Here's the drawing with two shaded views (mm, measured from the low corner). I have some questions. Coordinates: 2 decimals unless noted, no trailing zeros. Write each loop counter-clockwise with the first axis right and the second up, starting at its lowest first coordinate (ties: lowest second). Pieces come first, ordered by that corner, then holes. Notation, with made-up numbers: (51, -32) -> (75, -32) arc R31 ccw to (75, -7) -> close; hole circle Ø5 at (-19, -30). An arc over 180 degrees is marked (long way). Put each result on its own line as item: value. Start each with the question number.
Item 1: I need wall thicknesses on line 1 (Z direction, x = 6.35, y = 0.9); line 2 (X direction, y = 0.85, z = 107.95); line 3 (Z direction, x = 5.5, y = 1.3) (1 decimal). Which ranges of each line are inside material? Lowest first, please. Write a range as [from, to].
Item 2: I want a section at A-A, the plane x = 6.35. List the corners of the cut face in (y, z) for me.
Item 3: I want a section at B-B, the plane z = 107.95. List the corners of the cut face in (x, y) for me.
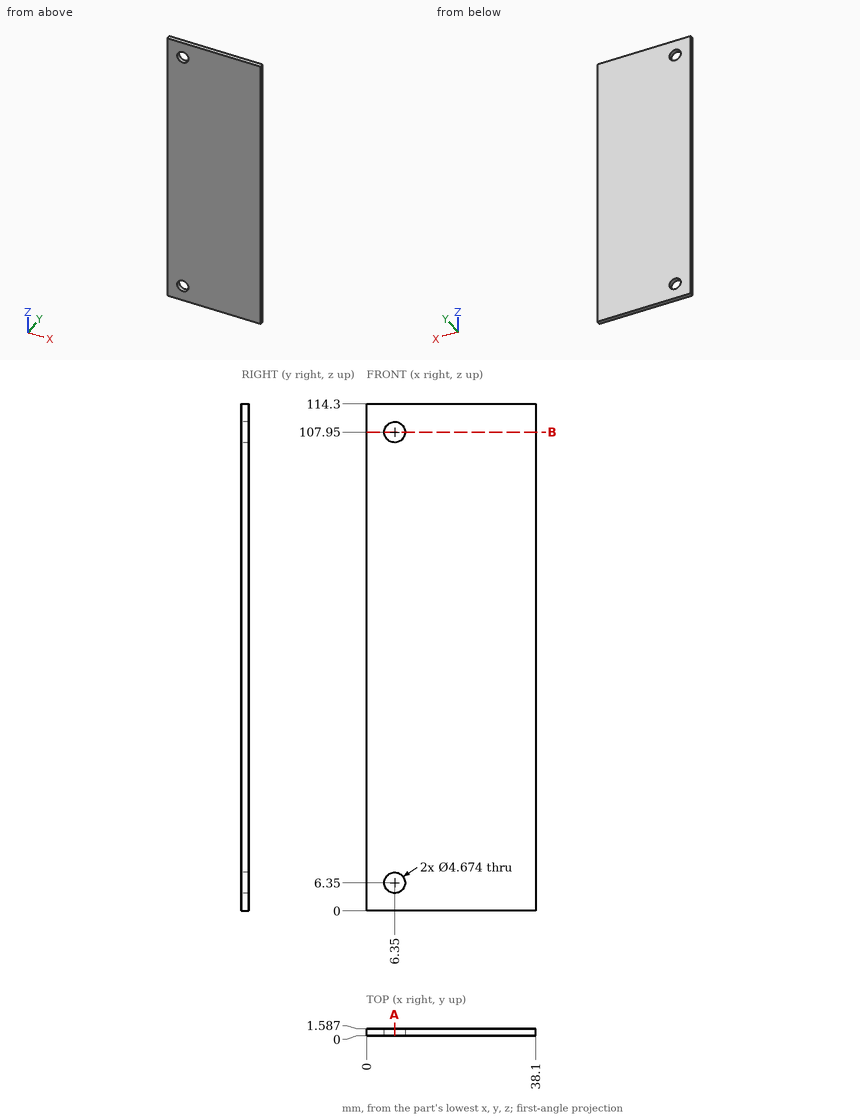
Calculated:
1. line 1: z = [0, 4.01], [8.69, 105.61], [110.29, 114.3]
1. line 2: x = [0, 4.01], [8.69, 38.1]
1. line 3: z = [0, 4.2], [8.5, 105.8], [110.1, 114.3]
2. outline: (0, 0) -> (1.59, 0) -> (1.59, 4.01) -> (0, 4.01) -> close; (0, 8.69) -> (1.59, 8.69) -> (1.59, 105.61) -> (0, 105.61) -> close; (0, 110.29) -> (1.59, 110.29) -> (1.59, 114.3) -> (0, 114.3) -> close
3. outline: (0, 0) -> (4.01, 0) -> (4.01, 1.59) -> (0, 1.59) -> close; (8.69, 0) -> (38.1, 0) -> (38.1, 1.59) -> (8.69, 1.59) -> close
